```python
from build123d import *

# Parameters (mm, degrees)
SKETCH3_W                = 114.3
SKETCH3_H                = 114.3
SKETCH3_R                = 5.55625
BOSS_EXTRUDE1_DEPTH      = 15.875
BOSS_EXTRUDE2_DEPTH      = 15.875
BOSS_EXTRUDE2_DEPTH_BACK = 15.875
SKETCH4_R                = 9.525


with BuildPart() as part:
    # Sketch3 → Boss-Extrude1 (new body)
    with BuildSketch(Plane.XY):
        Rectangle(SKETCH3_W, SKETCH3_H)
        with Locations((-42.2671875, -42.2671875)):
            Circle(SKETCH3_R, mode=Mode.SUBTRACT)
        with Locations((42.2671875, -42.2671875)):
            Circle(SKETCH3_R, mode=Mode.SUBTRACT)
        with Locations((42.2671875, 42.2671875)):
            Circle(SKETCH3_R, mode=Mode.SUBTRACT)
        with Locations((-42.2671875, 42.2671875)):
            Circle(SKETCH3_R, mode=Mode.SUBTRACT)
    extrude(amount=BOSS_EXTRUDE1_DEPTH)

    # Sketch4 → Boss-Extrude2 (add, two sides: drawn at the far end of the back side and taken through both)
    with BuildSketch(Plane(origin=(0, 0, 0), x_dir=(0, 0, -1), z_dir=(1, 0, 0)).offset(-BOSS_EXTRUDE2_DEPTH_BACK)):
        with BuildLine():
            Line((-48.400641314, 22.21146113), (-15.875, 23.347281553))
            Line((-15.875, 23.347281553), (-15.875, -23.347281553))
            Line((-15.875, -23.347281553), (-48.400641314, -22.21146113))
            ThreePointArc((-48.400641314, -22.21146113), (-69.85, 0), (-48.400641314, 22.21146113))
        make_face()
        with Locations((-47.625, 0)):
            Circle(SKETCH4_R, mode=Mode.SUBTRACT)
    extrude(amount=BOSS_EXTRUDE2_DEPTH + BOSS_EXTRUDE2_DEPTH_BACK)


solid = part.part
```
The model under review builds one solid part; all positions refer to its coordinate system, in mm. A direction names the side the tool comes from. Round coordinates to 2 decimals unless told otherwise and drop trailing zeros. Order: outer loops, then holes, each group sorted by start corner. A loop starts at its lowest first (then second) coordinate and runs counter-clockwise, first axis right, second up. Notation, with made-up numbers: M 36.25,66 L 54.25,66 A10 ccw 54.25,77 Z; hole C -12,84 d6. An arc over 180 degrees is marked long. Use a Markdown table: item, result.
1) Consider section C-C (z = 43.5). Write out the cut boundary in (x, y) (3 decimals), then the cut area to 3 significant figures.
Report:
| item | result |
|---|---|
| outline | M -15.875,-22.383 L 15.875,-22.383 L 15.875,-8.585 L -15.875,-8.585 Z; M -15.875,8.585 L 15.875,8.585 L 15.875,22.383 L -15.875,22.383 Z |
| area | 876 mm^2 |
2) Insertion check: pin 1 (6.5 mm diameter, centred on x = -42.27, y = 42.27, fed in from +Z); pin 2 (5 mm diameter, centred on x = 10, z = 20, fed in from -Y); pin 3 (14 mm diameter, centred on y = 8.5, z = 45.5, fed in from -X) (3 decimals); pin 4 (4 mm diameter, centred on x = -33, y = 0.5, fed in from +Z) (3 decimals). Each pin has a flat end and moves straight along its axis. Give the tip position at first contact, or say it passes through.
Report:
| item | result |
|---|---|
| pin 1 | through |
| pin 2 | y = -23.29 |
| pin 3 | x = -15.875 |
| pin 4 | z = 15.875 |
3) Wall thickness on line 1 along Z through (x, y) = (-47, -28) (3 decimals); line 2 along Y through (x, z) = (-1.5, 42); line 3 along X through (y, z) = (-8.5, 28.5) (3 decimals): over which ranges is each line inside the solid? List them lowest first. Write a range as [from, to].
Report:
| item | result |
|---|---|
| line 1 | [0, 15.875] |
| line 2 | [-22.43, -7.69], [7.69, 22.43] |
| line 3 | [-15.875, 15.875] |
4) Consider section A-A (x = -4). Write out the cut boundary in (y, z) (3 decimals).
Report:
| item | result |
|---|---|
| outline | M -57.15,0 L 57.15,0 L 57.15,15.875 L 23.347,15.875 L 22.211,48.401 A22.225 ccw -22.211,48.401 L -23.347,15.875 L -57.15,15.875 Z; hole C 0,47.625 d19.05 |
5) Draft analysis for pull direction X (two halves, no side actions). For faces 4 (the face through (-15.875, 0, 36)), 5 (the face through (-1, 1, 0)), 6 (the face through (-39.28, -37.58, 7.83)), state which applies: released by +X, released by -X, zero draft, split by the parting line, or undercut.
Report:
| item | result |
|---|---|
| face 4 | released by -X |
| face 5 | zero draft |
| face 6 | undercut |
6) Consider section B-B (y = 0). Write out the cut boundary in (x, z) (3 decimals), then the cut area to 3 significant figures.
Report:
| item | result |
|---|---|
| outline | M -57.15,0 L 57.15,0 L 57.15,15.875 L 15.875,15.875 L 15.875,38.1 L -15.875,38.1 L -15.875,15.875 L -57.15,15.875 Z; M -15.875,57.15 L 15.875,57.15 L 15.875,69.85 L -15.875,69.85 Z |
| area | 2,920 mm^2 |
7) Consider section D-D (x = -40). Write out the cut boundary in (y, z) (3 decimals), then the cut area to 3 significant figures.
Report:
| item | result |
|---|---|
| outline | M -57.15,0 L -47.34,0 L -47.34,15.875 L -57.15,15.875 Z; M -37.195,0 L 37.195,0 L 37.195,15.875 L -37.195,15.875 Z; M 47.34,0 L 57.15,0 L 57.15,15.875 L 47.34,15.875 Z |
| area | 1,490 mm^2 |
8) Tool access review of faces 1 (the face through (36.716, 42.511, 7.826)), 2 (the face through (15.875, 0, 36)), 3 (the face through (25, 1, 15.875)): name each direction out of +Z, -Z, +X, -X, +Y, -Y from which nothing blocks a thin tool from reaching the whole face with its end or side.
Report:
| item | result |
|---|---|
| face 1 | +Z, -Z |
| face 2 | +Z, +X, +Y, -Y |
| face 3 | +Z |
